Geometry check sheet. Reference: the model listing, model coordinates, mm. A direction names the side the tool comes from. Give positions to 0.01 mm unless a question says otherwise; leave off trailing zeros. Write each loop counter-clockwise with the first axis right and the second up, starting at its lowest first coordinate (ties: lowest second). Pieces come first, ordered by that corner, then holes.
(1) Cross-section at A-A (z = 29.5). Record the boundary of the cut face in (x, y).
(2) Depth check by flat-ended pin: P1, Ø3.5, axis at x = -0.5, z = 28, coming from the +Y side; P2, Ø0.7, axis at y = 0, z = 24, coming from the -X side; P3, Ø2, axis at x = -1, z = 46, coming from the -Y side. Enter the tip coordinate at first touch or a pass-through.
(3) Tool access check on faces 1 (the flat face through (0, 0.71, 36)), 2 (the flat face through (3.52, 0, 29)), 3 (the cylindrical face through (-0.29, 2.23, 5.57)), 4 (the flat face through (0, -0.71, 36)). Record the directions out of +Z, -Z, +X, -X, +Y, -Y that give a thin tool (end or side, any length) a straight path to the whole face; none if there is none.
(4) Cross-section at B-B (x = -6). Record the boundary of the cut face in (y, z).
(5) Thickness scan on line 1 along Z through (x, y) = (-3, -1); line 2 along Y through (x, z) = (-1, 19); line 3 along X through (y, z) = (0.25, 29.5). Record the ranges inside material, lowest first.
(6) Cross-section at C-C (z = 8.5). Record the boundary of the cut face in (x, y), and give its area (3 significant figures).
```python
from build123d import *

# Parameters (mm, degrees)
F0_R        = 2.25
F1_DEPTH    = 10
F2_W        = 17.2
F2_H        = 6.5
F2_R        = 2.25
F3_DEPTH    = 1.27
F4_W        = 7.04
F4_H        = 1.42
F5_DEPTH    = 50.8
F6_T1_DEPTH = 75.2661578682
F7_T1_DEPTH = 26.67
F8_R        = 1.27


# Not quite as in the source:
# - a fillet or chamfer that OpenCascade refuses, or shapes differently, is made with other operations: its cross-section is extruded or revolved along the edge and cut away or added


with BuildPart() as f1:
    # F0 (on Top) → F1 (new body)
    with BuildSketch(Plane.XY):
        Circle(F0_R)
    extrude(amount=F1_DEPTH)

    # F2 (on face) → F3 (join)
    with BuildSketch(Plane.XY.offset(10)):
        Rectangle(F2_W, F2_H)
        Circle(F2_R, mode=Mode.SUBTRACT)
        Circle(F2_R)
    extrude(amount=F3_DEPTH)

    # F4 (on face) → F5 (join)
    with BuildSketch(Plane.XY.offset(11.27)):
        Rectangle(F4_W, F4_H)
    extrude(amount=F5_DEPTH)

    # F6: chamfer of 3.81 x 14.2191135768 on 2 edges, made by hand

    # F6_s2 → F6_t1 (cut)
    with BuildSketch(Plane.XZ.offset(-37.6330789341)):
        Polygon((-3.52, 47.8508864232), (0.29, 62.07), (-3.52, 62.07), align=None)
        Polygon((3.52, 47.8508864232), (-0.29, 62.07), (3.52, 62.07), align=None)
    extrude(amount=F6_T1_DEPTH, mode=Mode.SUBTRACT)

    # F7: fillet of radius 5.08 on 4 edges, made by hand

    # F7_s2 → F7_t1 (cut)
    with BuildSketch(Plane.XY.offset(-2.7)):
        with BuildLine():
            ThreePointArc((-8.6, 1.83), (-7.1121024484, -1.7621024484), (-3.52, -3.25))
            Line((-3.52, -3.25), (-8.6, -3.25))
            Line((-8.6, -3.25), (-8.6, 1.83))
        make_face()
        with BuildLine():
            ThreePointArc((-3.52, 3.25), (-7.1121024484, 1.7621024484), (-8.6, -1.83))
            Line((-8.6, -1.83), (-8.6, 3.25))
            Line((-8.6, 3.25), (-3.52, 3.25))
        make_face()
        with BuildLine():
            ThreePointArc((8.6, 1.83), (7.1121024484, -1.7621024484), (3.52, -3.25))
            Line((3.52, -3.25), (8.6, -3.25))
            Line((8.6, -3.25), (8.6, 1.83))
        make_face()
        with BuildLine():
            ThreePointArc((3.52, 3.25), (7.1121024484, 1.7621024484), (8.6, -1.83))
            Line((8.6, -1.83), (8.6, 3.25))
            Line((8.6, 3.25), (3.52, 3.25))
        make_face()
    extrude(amount=F7_T1_DEPTH, mode=Mode.SUBTRACT)

    # F8
    f8_edges = [f1.edges().sort_by_distance(p)[0] for p in [
        (-2.25, 0, 0),
    ]]
    fillet(f8_edges, radius=F8_R)


solid = f1.part
```
Reply:
1. outline: (-3.52, -0.71) - (3.52, -0.71) - (3.52, 0.71) - (-3.52, 0.71) - close
2. P1: stops at y = 0.71
2. P2: stops at x = -3.52
2. P3: stops at y = -0.71
3. face 1: +Z, +X, -X, +Y
3. face 2: +Z, +X, +Y, -Y
3. face 3: -Z
3. face 4: +Z, +X, -X, -Y
4. outline: (-2.6, 10) - (2.6, 10) - (2.6, 11.27) - (-2.6, 11.27) - close
5. line 1: z = 10 to 11.27
5. line 2: y = -0.71 to 0.71
5. line 3: x = -3.52 to 3.52
6. outline: circle Ø4.5 at (0, 0)
6. area: 15.9 mm2
